Geometry check sheet. Reference: the model listing, model coordinates, mm. Face numbers are marked on the shaded views. A direction names the side the tool comes from. Give positions to 0.01 mm unless a question says otherwise; leave off trailing zeros. Order: outer loops, then holes, each group sorted by start corner. A loop starts at its lowest first (then second) coordinate and runs counter-clockwise, first axis right, second up. Notation, with made-up numbers: (44.25, 32) - (90.25, 32) arc R23 cw to (90.25, 49) - close; hole circle Ø2 at (87.5, -37.75). An arc over 180 degrees is marked (long way). Put each result on its own line as item: value. Start each with the question number.
```python
from build123d import *

# Parameters (mm, degrees)
SKETCH013_R     = 3.65
PAD006_DEPTH    = 4.62
SKETCH014_R     = 2.25
POCKET007_DEPTH = 2.2
SKETCH015_R     = 4.5
SKETCH015_R_2   = 2.9
POCKET008_DEPTH = 2.6
SKETCH016_R     = 4.5
SKETCH016_R_2   = 2.75
POCKET009_DEPTH = 1.6
FILLET004_R     = 0.2
FILLET005_R     = 0.3
FILLET006_R     = 0.3


with BuildPart() as part:
    # Sketch013 → Pad006 (new body)
    with BuildSketch(Plane.YZ):
        Circle(SKETCH013_R)
    extrude(amount=PAD006_DEPTH)

    # Sketch014 → Pocket007 (cut)
    with BuildSketch(Plane.YZ):
        Circle(SKETCH014_R)
    extrude(amount=POCKET007_DEPTH, mode=Mode.SUBTRACT)

    # Sketch015 → Pocket008 (cut)
    with BuildSketch(Plane.YZ):
        Circle(SKETCH015_R)
        Circle(SKETCH015_R_2, mode=Mode.SUBTRACT)
    extrude(amount=POCKET008_DEPTH, mode=Mode.SUBTRACT)

    # Sketch016 (on Face3 of Pocket008) → Pocket009 (cut)
    with BuildSketch(Plane.YZ.offset(4.62)):
        Circle(SKETCH016_R)
        Circle(SKETCH016_R_2, mode=Mode.SUBTRACT)
    extrude(amount=-POCKET009_DEPTH, mode=Mode.SUBTRACT)

    # Fillet004
    fillet004_edges = [part.edges().sort_by_distance(p)[0] for p in [
        (4.62, -2.75, 0),
    ]]
    fillet(fillet004_edges, radius=FILLET004_R)

    # Fillet005
    fillet005_edges = [part.edges().sort_by_distance(p)[0] for p in [
        (0, -2.25, 0),
        (0, -2.9, 0),
    ]]
    fillet(fillet005_edges, radius=FILLET005_R)

    # Fillet006
    fillet006_edges = [part.edges().sort_by_distance(p)[0] for p in [
        (2.2, -2.25, 0),
    ]]
    fillet(fillet006_edges, radius=FILLET006_R)


with BuildPart() as part_1:
    # Body002 placement: moved
    add(part.part.moved(Location((22, 6.35, 11.5))))


solid = part_1.part
```
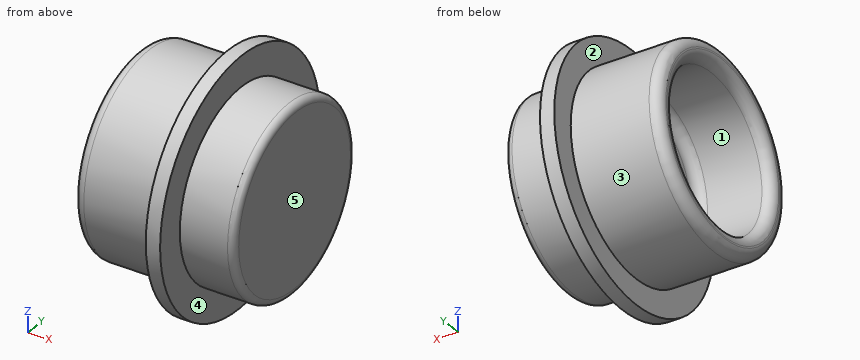
Item 1: Thickness scan on line 1 along Z through (x, y) = (23.35, 6.35); line 2 along X through (y, z) = (7, 11.5); line 3 along Z through (x, y) = (22.3, 5). Record the ranges inside material, lowest first.
Item 2: Gauge pin test, flat ends, axial feed: pin 1 Ø2 at (x, z) = (25.5, 13) entering from +Y; pin 2 Ø1.2 at (y, z) = (6.5, 11) entering from -X. Record the tip position at first contact, or that the pin passes through.
Item 3: Release check for a two-part mould opening along Z. For the marked faces 1, 2 and 3 record: +Z half, -Z half, draft (parallel to the pull), parting line (faces both ways), or undercut.
Item 4: Cross-section at C-C (x = 25.5). Enter the section's corners in (y, z), and give its area (3 significant figures).
Item 5: Cross-section at A-A (z = 11.5). Enter the section's corners in (x, y), and give its area (3 significant figures).
Item 6: Cross-section at D-D (x = 23.65). Enter the section's corners in (y, z), and give its area (3 significant figures).
Item 7: Cross-section at B-B (y = 6.35). Enter the section's corners in (x, z).
Item 8: Set-up check for the marked faces 4 and 5: record each of +Z, -Z, +X, -X, +Y, -Y from which the full face is reachable in a straight line by a thin tool's end or side.
Recorded:
1. line 1: z = 8.6 to 9.25, 13.75 to 14.4
1. line 2: x = 24.2 to 26.62
1. line 3: z = 8.93 to 9.7, 13.3 to 14.07
2. pin 1: stops at y = 9.95
2. pin 2: stops at x = 24.2
3. face 1: undercut
3. face 2: draft
3. face 3: parting line
4. outline: circle Ø5.5 at (6.35, 11.5)
4. area: 23.8 mm^2
5. outline: (22, 3.75) arc R0.3 ccw to (22.3, 3.45) - (24.6, 3.45) - (24.6, 2.7) - (25.02, 2.7) - (25.02, 3.6) - (26.42, 3.6) arc R0.2 ccw to (26.62, 3.8) - (26.62, 8.9) arc R0.2 ccw to (26.42, 9.1) - (25.02, 9.1) - (25.02, 10) - (24.6, 10) - (24.6, 9.25) - (22.3, 9.25) arc R0.3 ccw to (22, 8.95) - (22, 8.9) arc R0.3 ccw to (22.3, 8.6) - (23.9, 8.6) arc R0.3 cw to (24.2, 8.3) - (24.2, 4.4) arc R0.3 cw to (23.9, 4.1) - (22.3, 4.1) arc R0.3 ccw to (22, 3.8) - close
5. area: 17.0 mm^2
6. outline: circle Ø5.8 at (6.35, 11.5); hole circle Ø4.5 at (6.35, 11.5)
6. area: 10.5 mm^2
7. outline: (22, 8.9) arc R0.3 ccw to (22.3, 8.6) - (24.6, 8.6) - (24.6, 7.85) - (25.02, 7.85) - (25.02, 8.75) - (26.42, 8.75) arc R0.2 ccw to (26.62, 8.95) - (26.62, 14.05) arc R0.2 ccw to (26.42, 14.25) - (25.02, 14.25) - (25.02, 15.15) - (24.6, 15.15) - (24.6, 14.4) - (22.3, 14.4) arc R0.3 ccw to (22, 14.1) - (22, 14.05) arc R0.3 ccw to (22.3, 13.75) - (23.9, 13.75) arc R0.3 cw to (24.2, 13.45) - (24.2, 9.55) arc R0.3 cw to (23.9, 9.25) - (22.3, 9.25) arc R0.3 ccw to (22, 8.95) - close
8. face 4: +X
8. face 5: +Z, -Z, +X, +Y, -Y
